Source: CAD feature listing. Evaluate the final solid. Frame: model axes, mm. A direction names the side the tool comes from. Coordinates: 2 decimals unless noted, no trailing zeros. Order: outer loops, then holes, each group sorted by start corner. A loop starts at its lowest first (then second) coordinate and runs counter-clockwise, first axis right, second up.
```python
from build123d import *

# Parameters (mm, degrees)
BOSS_EXTRUDE1_DEPTH      = 10
BOSS_EXTRUDE1_DEPTH_BACK = 540
FILLET1_R                = 150
FILLET2_R                = 22.5
SHELL1_T                 = -4.5
CUT_EXTRUDE1_START       = -535
CUT_EXTRUDE1_DEPTH       = 79
SKETCH2_W                = 151.608609382
SKETCH2_H                = 22.921634695
BOSS_EXTRUDE2_DEPTH      = 50


with BuildPart() as part:
    # Sketch1 → Boss-Extrude1 (new, two sides: drawn at the far end of the back side and taken through both)
    with BuildSketch(Plane.XY.offset(-BOSS_EXTRUDE1_DEPTH_BACK)):
        Polygon((0, 0), (-780, 0), (-780, 900), (-540, 1110), (375, 1110), (825, 660), align=None)
    extrude(amount=BOSS_EXTRUDE1_DEPTH + BOSS_EXTRUDE1_DEPTH_BACK)

    # Fillet1
    fillet1_edges = [part.edges().sort_by_distance(p)[0] for p in [
        (-540, 1110, -265),
        (375, 1110, -265),
    ]]
    fillet(fillet1_edges, radius=FILLET1_R)

    # Fillet2
    fillet2_edges = [part.edges().sort_by_distance(p)[0] for p in [
        (621.966991411, 863.033008589, -540),
        (-85.38588347, 1110, -540),
        (-85.38588347, 1110, 10),
        (-681.207711882, 986.443252103, -540),
        (-536.398733566, 1100.415411602, -540),
        (370.270480499, 1098.581929877, -540),
        (-681.207711882, 986.443252103, 10),
        (-536.398733566, 1100.415411602, 10),
        (370.270480499, 1098.581929877, 10),
        (621.966991411, 863.033008589, 10),
    ]]
    fillet(fillet2_edges, radius=FILLET2_R)

    # Shell1
    shell1_openings = [part.faces().sort_by_distance(p)[0] for p in [
        (-390, 0, -265),
        (-780, 449.741271018, -265),
        (412.346232546, 329.876986037, -265),
    ]]
    offset(amount=SHELL1_T, openings=shell1_openings)

    # Sketch1<2> → Cut-Extrude1 (cut)
    with BuildSketch(Plane.XY.offset(CUT_EXTRUDE1_START)):
        Polygon((0, 0), (-780, 0), (-780, 900), (-540, 1110), (375, 1110), (825, 660), align=None)
    extrude(amount=-CUT_EXTRUDE1_DEPTH, mode=Mode.SUBTRACT)

    # Sketch2 → Boss-Extrude2 (add)
    with BuildSketch(Plane(origin=(0, 0, 5.5), x_dir=(-1, 0, 0), z_dir=(0, 0, -1))):
        with Locations((390, 11.460817348)):
            Rectangle(SKETCH2_W, SKETCH2_H)
    extrude(amount=BOSS_EXTRUDE2_DEPTH)


solid = part.part
```
1. Material intervals for line 1 along Y through (x, z) = (223, -342.5); line 2 along Z through (x, y) = (-329, 228); line 3 along X through (y, z) = (1040, -90.5), sorted ascending.
2. Access query for faces 1 (the flat face through (-682.591, 985.233, -268.535)), 2 (the flat face through (615.768, 862.868, -268.535)). Directions: +Z, -Z, +X, -X, +Y, -Y. A direction counts if a zero-diameter tool reaches every point of the face in a straight line with its end or side. Return the directions, or none.
3. Section query C-C, the plane y = 601. Output: boundary loops of the cut face in (x, z).
4. Section query D-D, the plane x = 86. Output: boundary loops of the cut face in (y, z).
5. Section query A-A, the plane x = -431. Output: boundary loops of the cut face in (y, z), plus the area to 3 significant figures.
6. Section query B-B, the plane z = -415. Output: boundary loops of the cut face in (x, y), plus the area to 3 significant figures.
7. Draft query along Z for faces 3 (the cylindrical face through (620.03, 855.41, 3.58)), 4 (the cylindrical face through (617.62, 853.36, 0.37)), 5 (the flat face through (-91, 1110, -269)). Return one class per face: +Z half, -Z half, draft (parallel to the pull), parting line (faces both ways), or undercut.
8. Contact query for flat-ended pins moving along their axis: P1, Ø10, axis at y = 741, z = -448, coming from the -X side; P2, Ø11.5, axis at x = -396.5, y = 7.5, coming from the -Z side; P3, Ø7, axis at y = 9.5, z = -13, coming from the -X side. Output: stop coordinate, or through.
Answer key:
1. line 1: y = 1105.5 to 1110
1. line 2: z = 5.5 to 10
1. line 3: x = -620 to -613.17, 438.64 to 445
2. face 1: +Z, -Z, -X, +Y
2. face 2: -Y
3. outline: (-780, 5.5) - (751.25, 5.5) - (751.25, 10) - (-780, 10) - close
4. outline: (68.8, 5.5) - (1087.5, 5.5) arc R18 cw to (1105.5, -12.5) - (1105.5, -517.5) arc R18 cw to (1091.71, -535) - (1101.64, -535) arc R22.5 ccw to (1110, -517.5) - (1110, -12.5) arc R22.5 ccw to (1087.5, 10) - (68.8, 10) - close
5. outline: (0, -44.5) - (22.92, -44.5) - (22.92, 5.5) - (1087.5, 5.5) arc R18 cw to (1105.5, -12.5) - (1105.5, -517.5) arc R18 cw to (1091.71, -535) - (1101.64, -535) arc R22.5 ccw to (1110, -517.5) - (1110, -12.5) arc R22.5 ccw to (1087.5, 10) - (0, 10) - close
5. area: 8,550 mm2
6. outline: (-780, 894.02) - (-579.45, 1069.5) arc R145.5 cw to (-483.64, 1105.5) - (312.87, 1105.5) arc R145.5 cw to (415.75, 1062.88) - (821.46, 657.17) - (825, 660) - (418.93, 1066.07) arc R150 ccw to (312.87, 1110) - (-483.64, 1110) arc R150 ccw to (-582.42, 1072.89) - (-780, 900) - close
6. area: 8,360 mm2
7. face 3: +Z half
7. face 4: undercut
7. face 5: draft
8. P1: stops at x = 732.64
8. P2: stops at z = -44.5
8. P3: stops at x = -465.8
